```python
from build123d import *

# Parameters (mm, degrees)
SKETCH014_R      = 12
EXTRUDE006_DEPTH = 150
EXTRUDE005_DEPTH = 30
SKETCH012_W      = 15
SKETCH012_H      = 79.05159
SKETCH012_H_2    = 80
EXTRUDE004_DEPTH = 150


with BuildPart() as extrude006:
    # Sketch014 → Extrude006 (new body, symmetric)
    with BuildSketch(Plane.YZ):
        Circle(SKETCH014_R)
    extrude(amount=EXTRUDE006_DEPTH, both=True)


with BuildPart() as extrude005:
    # Sketch013 → Extrude005 (new body, symmetric)
    with BuildSketch(Plane.XZ):
        with BuildLine():
            Line((62, 10), (62, -10))
            ThreePointArc((57, -15), (60.535534, -13.535534), (62, -10))
            Line((57, -15), (-57, -15))
            ThreePointArc((-62, -10), (-60.535534, -13.535534), (-57, -15))
            Line((-62, -10), (-62, 10))
            ThreePointArc((-57, 15), (-60.535534, 13.535534), (-62, 10))
            Line((-57, 15), (57, 15))
            ThreePointArc((62, 10), (60.535534, 13.535534), (57, 15))
        make_face()
    extrude(amount=EXTRUDE005_DEPTH, both=True)


with BuildPart() as extrude004:
    # Sketch012 → Extrude004 (new body, symmetric)
    with BuildSketch(Plane.YZ):
        with Locations((-28.5, 0.159191)):
            Rectangle(SKETCH012_W, SKETCH012_H)
        with Locations((28.5, -0.315014)):
            Rectangle(SKETCH012_W, SKETCH012_H_2)
    extrude(amount=EXTRUDE004_DEPTH, both=True)


with BuildPart() as obj1:
    # Sketch011 → Revolve (revolve)
    with BuildSketch(Plane.XZ):
        Polygon((-100, 0), (-100, 21), (-62, 27), (62, 27), (100, 21), (100, 0), align=None)
    revolve(axis=Axis((-100, 0, 0), (-1, 0, 0)))

    # Cut004: cut Extrude004
    add(extrude004.part, mode=Mode.SUBTRACT)

    # Cut005: cut Extrude005
    add(extrude005.part, mode=Mode.SUBTRACT)

    # Cut006: cut Extrude006
    add(extrude006.part, mode=Mode.SUBTRACT)


with BuildPart() as obj1_1:
    # Cut006 placement: moved
    add(obj1.part.moved(Location((-404, 0, 0))))


solid = obj1_1.part
```
Verification items for the finished model (mm, model axes). A direction names the side the tool comes from. Give positions to 0.01 mm unless a question says otherwise; leave off trailing zeros. Order: outer loops, then holes, each group sorted by start corner. A loop starts at its lowest first (then second) coordinate and runs counter-clockwise, first axis right, second up. Notation, with made-up numbers: M 28,89.5 L 82,89.5 A13 cw 82,97.5 Z; hole C 48.5,86.25 d2. An arc over 180 degrees is marked long. Answer in a Markdown table with one row per item. Add a question column.
Item 1: Scan lines: probe 1 along X at (y, z) = (-13, 3); probe 2 along Y at (x, z) = (-320, 0); probe 3 along Z at (x, y) = (-494, 0). Record each from-to range of solid material in increasing order. Write a range as from..to.
Item 2: Gauge pin test, flat ends, axial feed: pin 1 (12 mm diameter, centred on x = -456.5, y = -12, fed in from +Z); pin 2 (6 mm diameter, centred on x = -361.5, y = 12, fed in from +Z). Record the tip position at first contact, or that the pin passes through.
Item 3: Section check B-B, the plane y = 0. Enter the section's corners in (x, z), and give its area (3 significant figures).
Item 4: Mould release check, pull along Z, two halves, no side actions. Record for faces 1 (the flat face through (-402.6, 21, -15.3)), 2 (the cylindrical face through (-322.94, -11.99, 0.53)), 3 (the cylindrical face through (-344, 0, -14)), 4 (the conical face through (-488.96, 0.51, -23.37)): released by +Z, released by -Z, zero draft, split by the parting line, or undercut.
Item 5: Section check A-A, the plane x = -374. Enter the section's corners in (y, z), and give its area (3 significant figures).
Item 6: Section check C-C, the plane z = 6. State how many separate pieces and enclosed holes the cut face has, and give its area (3 significant figures).
Item 7: Tool access check on faces 5 (the cylindrical face through (-484.52, -11.99, 0.53)), 6 (the flat face through (-403, 0, -15)). Record the directions out of +Z, -Z, +X, -X, +Y, -Y that give a thin tool (end or side, any length) a straight path to the whole face; none if there is none.
Filled sheet:
| question | item | result |
|---|---|---|
| 1 | probe 1 | x = -504..-466, -342..-304 |
| 1 | probe 2 | y = -21..-12, 12..21 |
| 1 | probe 3 | z = -22.58..-12, 12..22.58 |
| 2 | pin 1 | stops at z = 26.32 |
| 2 | pin 2 | stops at z = 25.46 |
| 3 | outline | M -504,-21 L -466,-27 L -342,-27 L -304,-21 L -304,-12 L -342.42,-12 A5 cw -347,-15 L -461,-15 A5 cw -465.58,-12 L -504,-12 Z; M -504,12 L -465.58,12 A5 cw -461,15 L -347,15 A5 cw -342.42,12 L -304,12 L -304,21 L -342,27 L -466,27 L -504,21 Z |
| 3 | area | 4,820 mm^2 |
| 4 | face 1 | zero draft |
| 4 | face 2 | undercut |
| 4 | face 3 | undercut |
| 4 | face 4 | released by -Z |
| 5 | outline | M -21,-16.97 A27 ccw 21,-16.97 L 21,-15 L -21,-15 Z; M -21,15 L 21,15 L 21,16.97 A27 ccw -21,16.97 Z |
| 5 | area | 752 mm^2 |
| 6 | separate pieces | 4 |
| 6 | enclosed holes | 0 |
| 6 | area | 1,600 mm^2 |
| 7 | face 5 | +X, -X |
| 7 | face 6 | +Y, -Y |
